```python
from build123d import *

# Parameters (mm, degrees)
F0_W     = 50.8
F0_H     = 50.8
F1_DEPTH = 51.054
F2_R     = 14.677171
F3_DEPTH = 43.688
F5_DEPTH = 25.4
F6_DEPTH = 25.4


with BuildPart() as f1:
    # F0 (on Top) → F1 (new body)
    with BuildSketch(Plane.XY):
        Rectangle(F0_W, F0_H)
    extrude(amount=F1_DEPTH)

    # F2 (on face) → F3 (join)
    with BuildSketch(Plane.XY.offset(51.054)):
        Circle(F2_R)
    extrude(amount=F3_DEPTH)

    # F4 (on Front) → F5 (cut)
    with BuildSketch(Plane.XZ):
        Polygon((-17.87798, 85.614286), (-14.499731, 85.614286), (14.499732, 69.13732), (21.090519, 95.280774), (-17.35574, 97.038314), align=None)
    extrude(amount=F5_DEPTH, mode=Mode.SUBTRACT)

    # F4 (on Front) → F6 (cut)
    with BuildSketch(Plane.XZ):
        Polygon((-17.87798, 85.614286), (-14.499731, 85.614286), (14.499732, 69.13732), (21.090519, 95.280774), (-17.35574, 97.038314), align=None)
    extrude(amount=-F6_DEPTH, mode=Mode.SUBTRACT)


solid = f1.part
```
The listing builds one solid part. Answer for the finished solid, in the listing's coordinates (mm). A direction names the side the tool comes from. Round coordinates to 2 decimals unless told otherwise and drop trailing zeros. Loops run counter-clockwise (first coordinate to the right, second up) from the corner with the lowest first, then second, coordinate; pieces in that order, holes last.
Q1. Section B-B, the plane x = 0 is taken. Determine the outline of the cut face in (y, z).
Q2. Find the intervals of material crossed by line 1 (Z direction, x = -14.5, y = -8.5); line 2 (Y direction, x = -3, z = 61); line 3 (X direction, y = -9, z = 74.5), in increasing order.
Q3. Section D-D, the plane y = -18.5 is taken. Determine the outline of the cut face in (x, z).
Q4. Section A-A, the plane y = 0 is taken. Determine the outline of the cut face in (x, z).
Q5. Which of the six approach directions +Z, -Z, +X, -X, +Y, -Y give full straight-line access (tool end or side, diameter ignored) to faces 1 (the face through (11, -11, 51.054)), 2 (the face through (0, 0, 0))?
Q6. Section C-C, the plane x = 8.5 is taken. Determine the outline of the cut face in (y, z).
Q7. Given pin 1 Ø5 at (x, y) = (-2.5, 0) entering from +Z; pin 2 Ø1 at (x, y) = (10.5, -17.5) entering from +Z; pin 3 Ø5 at (y, z) = (-12, 76) entering from -X, each flat-ended and moving along its own axis, determine where each tip first touches the part or whether it passes through.
Completed:
1. outline: (-25.4, 0) - (25.4, 0) - (25.4, 51.05) - (14.68, 51.05) - (14.68, 77.38) - (-14.68, 77.38) - (-14.68, 51.05) - (-25.4, 51.05) - close
2. line 1: z = 0 to 51.05
2. line 2: y = -14.37 to 14.37
2. line 3: x = -11.59 to 5.06
3. outline: (-25.4, 0) - (25.4, 0) - (25.4, 51.05) - (-25.4, 51.05) - close
4. outline: (-25.4, 0) - (25.4, 0) - (25.4, 51.05) - (14.68, 51.05) - (14.68, 69.84) - (14.5, 69.14) - (-14.5, 85.61) - (-14.68, 85.61) - (-14.68, 51.05) - (-25.4, 51.05) - close
5. face 1: +Z
5. face 2: -Z, +X, -X, +Y, -Y
6. outline: (-25.4, 0) - (25.4, 0) - (25.4, 51.05) - (11.97, 51.05) - (11.97, 72.55) - (-11.97, 72.55) - (-11.97, 51.05) - (-25.4, 51.05) - close
7. pin 1: stops at z = 80.22
7. pin 2: stops at z = 51.05
7. pin 3: stops at x = -11.19
